Input: part model. Units: mm. Frame: model coordinates. Face numbers are marked on the shaded views. Coordinates: 2 decimals unless noted, no trailing zeros. Use a Markdown table: item, result. Add a question column.
1. Draft query along Z for the marked faces 1 and 2. Return one class per face: released by +Z, released by -Z, zero draft, split by the parting line, or undercut.
2. Section query A-A on x = -63. State how many separate pieces and enclosed holes the cut face has, then the cut area to 3 significant figures.
3. Ray query, L1, parallel to Y at x = -117.5, z = 1.65; L2, parallel to Y at x = -39.5, z = 3.2; L3, parallel to X at y = 98.5, z = 0.95. Return the intervals inside material, ascending. Write a range as [from, to].
4. Contact query for a flat-ended pin moving along its axis: P1, Ø6.5, axis at x = -38.59, y = 102.91, coming from the -Z side. Output: stop coordinate, or through.
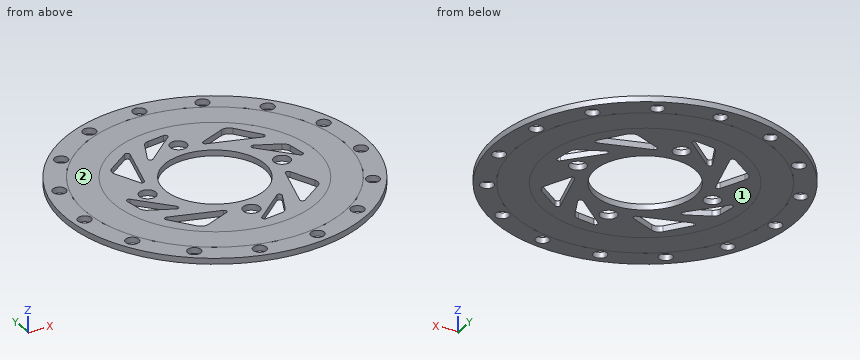
```python
from build123d import *

# Parameters (mm, degrees)
SKETCH1_R                = 90
SKETCH1_R_2              = 30
SKETCH1_R_3              = 5
SKETCH1_R_4              = 4
SKETCH1_R_5              = 4.163878313
BOSS_EXTRUDE1_DEPTH      = 3.5
SKETCH3_R                = 77.611648898
SKETCH3_R_2              = 60.616629638
BOSS_EXTRUDE2_DEPTH      = 0.001
BOSS_EXTRUDE2_DEPTH_BACK = 3.501


with BuildPart() as part:
    # Sketch1 → Boss-Extrude1 (new body)
    with BuildSketch(Plane.XY):
        with Locations((-38.590160458, 20.233035518)):
            Circle(SKETCH1_R)
        with Locations((-38.590160458, 20.233035518)):
            Circle(SKETCH1_R_2, mode=Mode.SUBTRACT)
        with Locations((-38.590160458, 60.233035518)):
            Circle(SKETCH1_R_3, mode=Mode.SUBTRACT)
        with Locations((-78.590160458, 20.233035518)):
            Circle(SKETCH1_R_3, mode=Mode.SUBTRACT)
        with Locations((-38.590160458, -19.766964482)):
            Circle(SKETCH1_R_3, mode=Mode.SUBTRACT)
        with Locations((1.409839542, 20.233035518)):
            Circle(SKETCH1_R_3, mode=Mode.SUBTRACT)
        with Locations((-38.590160458, 102.908863271)):
            Circle(SKETCH1_R_4, mode=Mode.SUBTRACT)
        with Locations((-57.272235988, 84.226787741)):
            Circle(SKETCH1_R_5, mode=Mode.SUBTRACT)
        with Locations((-47.931198223, 93.567825506)):
            Circle(SKETCH1_R_4, mode=Mode.SUBTRACT)
        with Locations((-29.628481741, 86.292921865)):
            Circle(SKETCH1_R_5, mode=Mode.SUBTRACT)
        with Locations((-17.295676778, 91.027042142)):
            Circle(SKETCH1_R_4, mode=Mode.SUBTRACT)
        with Locations((-4.962871814, 95.761162419)):
            Circle(SKETCH1_R_4, mode=Mode.SUBTRACT)
        with Locations((-3.534283159, 76.936701505)):
            Circle(SKETCH1_R_5, mode=Mode.SUBTRACT)
        with Locations((9.657834985, 76.24533189)):
            Circle(SKETCH1_R_4, mode=Mode.SUBTRACT)
        with Locations((22.849953128, 75.553962274)):
            Circle(SKETCH1_R_4, mode=Mode.SUBTRACT)
        with Locations((16.498435766, 57.77590216)):
            Circle(SKETCH1_R_5, mode=Mode.SUBTRACT)
        with Locations((28.268830016, 51.778586739)):
            Circle(SKETCH1_R_4, mode=Mode.SUBTRACT)
        with Locations((40.039224266, 45.781271318)):
            Circle(SKETCH1_R_4, mode=Mode.SUBTRACT)
        with Locations((27.00583594, 32.123600105)):
            Circle(SKETCH1_R_5, mode=Mode.SUBTRACT)
        with Locations((35.3192982, 21.857329199)):
            Circle(SKETCH1_R_4, mode=Mode.SUBTRACT)
        with Locations((43.63276046, 11.591058294)):
            Circle(SKETCH1_R_4, mode=Mode.SUBTRACT)
        with Locations((26.171092415, 4.415311411)):
            Circle(SKETCH1_R_5, mode=Mode.SUBTRACT)
        with Locations((29.590149535, -8.344783474)):
            Circle(SKETCH1_R_4, mode=Mode.SUBTRACT)
        with Locations((33.009206655, -21.104878358)):
            Circle(SKETCH1_R_4, mode=Mode.SUBTRACT)
        with Locations((14.138539931, -20.557949085)):
            Circle(SKETCH1_R_5, mode=Mode.SUBTRACT)
        with Locations((12.072005874, -33.605531622)):
            Circle(SKETCH1_R_4, mode=Mode.SUBTRACT)
        with Locations((10.005471816, -46.653114158)):
            Circle(SKETCH1_R_4, mode=Mode.SUBTRACT)
        with Locations((-7.011283875, -38.478077769)):
            Circle(SKETCH1_R_5, mode=Mode.SUBTRACT)
        with Locations((-14.206086598, -49.557102403)):
            Circle(SKETCH1_R_4, mode=Mode.SUBTRACT)
        with Locations((-21.40088932, -60.636127037)):
            Circle(SKETCH1_R_4, mode=Mode.SUBTRACT)
        with Locations((-33.621382328, -46.246521592)):
            Circle(SKETCH1_R_5, mode=Mode.SUBTRACT)
        with Locations((-44.700406962, -53.441324315)):
            Circle(SKETCH1_R_4, mode=Mode.SUBTRACT)
        with Locations((-55.779431596, -60.636127037)):
            Circle(SKETCH1_R_4, mode=Mode.SUBTRACT)
        with Locations((-61.090627659, -42.520046043)):
            Circle(SKETCH1_R_5, mode=Mode.SUBTRACT)
        with Locations((-74.138210196, -44.5865801)):
            Circle(SKETCH1_R_4, mode=Mode.SUBTRACT)
        with Locations((-87.185792732, -46.653114158)):
            Circle(SKETCH1_R_4, mode=Mode.SUBTRACT)
        with Locations((-84.669337801, -27.942992598)):
            Circle(SKETCH1_R_5, mode=Mode.SUBTRACT)
        with Locations((-97.429432686, -24.523935478)):
            Circle(SKETCH1_R_4, mode=Mode.SUBTRACT)
        with Locations((-110.189527571, -21.104878358)):
            Circle(SKETCH1_R_4, mode=Mode.SUBTRACT)
        with Locations((-100.280539565, -5.035866226)):
            Circle(SKETCH1_R_5, mode=Mode.SUBTRACT)
        with Locations((-110.54681047, 3.277596034)):
            Circle(SKETCH1_R_4, mode=Mode.SUBTRACT)
        with Locations((-120.813081376, 11.591058294)):
            Circle(SKETCH1_R_4, mode=Mode.SUBTRACT)
        with Locations((-105.224914341, 22.240482818)):
            Circle(SKETCH1_R_5, mode=Mode.SUBTRACT)
        with Locations((-111.222229762, 34.010877068)):
            Circle(SKETCH1_R_4, mode=Mode.SUBTRACT)
        with Locations((-117.219545183, 45.781271318)):
            Circle(SKETCH1_R_4, mode=Mode.SUBTRACT)
        with Locations((-98.647534813, 49.169725987)):
            Circle(SKETCH1_R_5, mode=Mode.SUBTRACT)
        with Locations((-99.338904429, 62.36184413)):
            Circle(SKETCH1_R_4, mode=Mode.SUBTRACT)
        with Locations((-100.030274045, 75.553962274)):
            Circle(SKETCH1_R_4, mode=Mode.SUBTRACT)
        with Locations((-81.685689655, 71.095552492)):
            Circle(SKETCH1_R_5, mode=Mode.SUBTRACT)
        with Locations((-76.951569379, 83.428357455)):
            Circle(SKETCH1_R_4, mode=Mode.SUBTRACT)
        with Locations((-72.217449102, 95.761162419)):
            Circle(SKETCH1_R_4, mode=Mode.SUBTRACT)
        with BuildLine():
            Line((-75.923250233, 33.526611773), (-82.945064437, 48.18024702))
            ThreePointArc((-82.945064437, 48.18024702), (-83.308109154, 51.464629536), (-81.543225165, 54.258221219))
            Line((-81.543225165, 54.258221219), (-67.922632883, 65.062083457))
            ThreePointArc((-67.922632883, 65.062083457), (-66.174715863, 65.145679261), (-65.537023858, 63.516093095))
            Line((-65.537023858, 63.516093095), (-73.117089427, 33.80401367))
            ThreePointArc((-73.117089427, 33.80401367), (-74.422973645, 32.682089003), (-75.923250233, 33.526611773))
        make_face(mode=Mode.SUBTRACT)
        with BuildLine():
            Line((-25.019182306, 54.759964487), (4.692897118, 47.179898918))
            ThreePointArc((4.692897118, 47.179898918), (6.322483285, 47.817590922), (6.238887481, 49.565507943))
            Line((6.238887481, 49.565507943), (-4.564974758, 63.186100225))
            ThreePointArc((-4.564974758, 63.186100225), (-7.35856644, 64.950984214), (-10.642948957, 64.587939497))
            Line((-10.642948957, 64.587939497), (-25.296584204, 57.566125293))
            ThreePointArc((-25.296584204, 57.566125293), (-26.141106973, 56.065848705), (-25.019182306, 54.759964487))
        make_face(mode=Mode.SUBTRACT)
        with BuildLine():
            Line((-4.06323149, 6.662057366), (-11.643297059, -23.050022058))
            ThreePointArc((-11.643297059, -23.050022058), (-11.005605054, -24.679608225), (-9.257688034, -24.596012421))
            Line((-9.257688034, -24.596012421), (4.362904249, -13.792150183))
            ThreePointArc((4.362904249, -13.792150183), (6.127788237, -10.9985585), (5.764743521, -7.714175984))
            Line((5.764743521, -7.714175984), (-1.257070683, 6.939459263))
            ThreePointArc((-1.257070683, 6.939459263), (-2.757347272, 7.783982033), (-4.06323149, 6.662057366))
        make_face(mode=Mode.SUBTRACT)
        with BuildLine():
            Line((-52.16113861, -14.29389345), (-81.873218035, -6.713827882))
            ThreePointArc((-81.873218035, -6.713827882), (-83.502804202, -7.351519886), (-83.419208397, -9.099436907))
            Line((-83.419208397, -9.099436907), (-72.615346159, -22.720029189))
            ThreePointArc((-72.615346159, -22.720029189), (-69.821754476, -24.484913178), (-66.53737196, -24.121868461))
            Line((-66.53737196, -24.121868461), (-51.883736713, -17.100054257))
            ThreePointArc((-51.883736713, -17.100054257), (-51.039213944, -15.599777669), (-52.16113861, -14.29389345))
        make_face(mode=Mode.SUBTRACT)
        with BuildLine():
            Line((-50.430809264, 71.604828983), (-40.306353074, 73.454044222))
            ThreePointArc((-40.306353074, 73.454044222), (-38.700938161, 72.66063457), (-38.999542003, 70.894935936))
            Line((-38.999542003, 70.894935936), (-57.510335459, 53.1738017))
            ThreePointArc((-57.510335459, 53.1738017), (-59.397534082, 53.021332689), (-59.930645054, 54.838076517))
            Line((-59.930645054, 54.838076517), (-54.14247101, 68.622050752))
            ThreePointArc((-54.14247101, 68.622050752), (-52.664508346, 70.58364545), (-50.430809264, 71.604828983))
        make_face(mode=Mode.SUBTRACT)
        with BuildLine():
            Line((12.781633006, 32.073684324), (14.630848245, 21.949228134))
            ThreePointArc((14.630848245, 21.949228134), (13.837438594, 20.34381322), (12.07173996, 20.642417062))
            Line((12.07173996, 20.642417062), (-5.649394276, 39.153210519))
            ThreePointArc((-5.649394276, 39.153210519), (-5.801863288, 41.040409142), (-3.98511946, 41.573520114))
            Line((-3.98511946, 41.573520114), (9.798854776, 35.78534607))
            ThreePointArc((9.798854776, 35.78534607), (11.760449474, 34.307383406), (12.781633006, 32.073684324))
        make_face(mode=Mode.SUBTRACT)
        with BuildLine():
            Line((-26.749511652, -31.138757947), (-36.873967842, -32.987973185))
            ThreePointArc((-36.873967842, -32.987973185), (-38.479382756, -32.194563534), (-38.180778914, -30.4288649))
            Line((-38.180778914, -30.4288649), (-19.669985458, -12.707730664))
            ThreePointArc((-19.669985458, -12.707730664), (-17.782786834, -12.555261653), (-17.249675862, -14.372005481))
            Line((-17.249675862, -14.372005481), (-23.037849906, -28.155979716))
            ThreePointArc((-23.037849906, -28.155979716), (-24.51581257, -30.117574414), (-26.749511652, -31.138757947))
        make_face(mode=Mode.SUBTRACT)
        with BuildLine():
            Line((-89.961953923, 8.392386712), (-91.811169162, 18.516842902))
            ThreePointArc((-91.811169162, 18.516842902), (-91.01775951, 20.122257816), (-89.252060876, 19.823653974))
            Line((-89.252060876, 19.823653974), (-71.53092664, 1.312860518))
            ThreePointArc((-71.53092664, 1.312860518), (-71.378457629, -0.574338106), (-73.195201457, -1.107449078))
            Line((-73.195201457, -1.107449078), (-86.979175693, 4.680724966))
            ThreePointArc((-86.979175693, 4.680724966), (-88.940770391, 6.15868763), (-89.961953923, 8.392386712))
        make_face(mode=Mode.SUBTRACT)
    extrude(amount=BOSS_EXTRUDE1_DEPTH)

    # Sketch3 → Boss-Extrude2 (add, two sides)
    with BuildSketch(Plane(origin=(0, 0, 0), x_dir=(-1, 0, 0), z_dir=(0, 0, -1))) as boss_extrude2_sk:
        with Locations((38.590160458, 20.233035518)):
            Circle(SKETCH3_R)
        with Locations((38.590160458, 20.233035518)):
            Circle(SKETCH3_R_2, mode=Mode.SUBTRACT)
    extrude(amount=BOSS_EXTRUDE2_DEPTH)
    extrude(boss_extrude2_sk.sketch, amount=-BOSS_EXTRUDE2_DEPTH_BACK)


solid = part.part
```
Resolved:
| question | item | result |
|---|---|---|
| 1 | face 1 | released by -Z |
| 1 | face 2 | released by +Z |
| 2 | separate pieces | 3 |
| 2 | enclosed holes | 0 |
| 2 | area | 446 mm² |
| 3 | L1 | [-23.05, 9.35], [13.83, 41.79], [49.77, 63.51] |
| 3 | L2 | [-69.76, -24.68], [-14.85, -9.75], [50.22, 55.32], [65.15, 70.42], [73.38, 99.01], [106.8, 110.23] |
| 3 | L3 | [-83.02, -75.13], [-69.3, -7.88], [-2.05, 5.84] |
| 4 | P1 | through |
